Work out the finished part from the listing and answer in its coordinate system (mm). A direction names the side the tool comes from. Round coordinates to 2 decimals unless told otherwise and drop trailing zeros. Order: outer loops, then holes, each group sorted by start corner. A loop starts at its lowest first (then second) coordinate and runs counter-clockwise, first axis right, second up. Notation, with made-up numbers: M 2,-2 L 47,-2 A16 ccw 47,19 Z; hole C -1.5,-35.5 d1. An arc over 180 degrees is marked long. Return JSON: item names as keys, results as strings.
from build123d import *

# Parameters (mm, degrees)
SKETCH1_W                             = 160.4
SKETCH1_H                             = 40
SKETCH1_R                             = 9.5
BOSS_EXTRUDE1_DEPTH                   = 5
TAP_DRILL_FOR_M5_HELICOIL1_AT_2_COUNT = 2
TAP_DRILL_FOR_M5_HELICOIL1_AT_2_PITCH = 20
FILLET1_R                             = 3
M5_CLEARANCE_HOLE1_D                  = 5.5


with BuildPart() as part:
    # Sketch1 → Boss-Extrude1 (new body, symmetric)
    with BuildSketch(Plane(origin=(0, 0, 0), x_dir=(1, 0, 0), z_dir=(0, 1, 0))):
        Rectangle(SKETCH1_W, SKETCH1_H)
        Circle(SKETCH1_R, mode=Mode.SUBTRACT)
    extrude(amount=BOSS_EXTRUDE1_DEPTH, both=True)

    # Sketch4 → Tap Drill for M5 Helicoil1 (revolve, cut)
    with BuildSketch(Plane(origin=(-80.2, 0, -10), x_dir=(0, 0, 1), z_dir=(0, 1, 0))):
        Polygon((0, 0), (0, 31.562237609), (2.6, 30), (2.6, 0), align=None)
    tap_drill_for_m5_helicoil1 = revolve(axis=Axis((-86.55, 0, -10), (1, 0, 0)), mode=Mode.SUBTRACT)

    # Tap Drill for M5 Helicoil1 at 2: Tap Drill for M5 Helicoil1 ×2
    with Locations(*[(0, 0, i * TAP_DRILL_FOR_M5_HELICOIL1_AT_2_PITCH) for i in range(1, TAP_DRILL_FOR_M5_HELICOIL1_AT_2_COUNT)]):
        add(tap_drill_for_m5_helicoil1, mode=Mode.SUBTRACT)

    # Mirror1: Tap Drill for M5 Helicoil1 across plane
    add(tap_drill_for_m5_helicoil1.mirror(Plane(origin=(0, 0, 0), x_dir=(0, 0, 1), z_dir=(1, 0, 0))), mode=Mode.SUBTRACT)

    # Mirror1 copy 1 sketch → Mirror1 copy 1 (revolve, cut)
    with BuildSketch(Plane(origin=(80.2, 0, 10), x_dir=(0, 0, 1), z_dir=(0, 1, 0))):
        Polygon((0, 0), (0, -31.562237609), (2.6, -30), (2.6, 0), align=None)
    revolve(axis=Axis((86.55, 0, 10), (1, 0, 0)), mode=Mode.SUBTRACT)

    # Fillet1
    fillet1_edges = [part.edges().sort_by_distance(p)[0] for p in [
        (-80.2, 0, -20),
        (80.2, 0, -20),
        (80.2, 0, 20),
        (-80.2, 0, 20),
    ]]
    fillet(fillet1_edges, radius=FILLET1_R)

    # M5 Clearance Hole1 (through all)
    with Locations(Plane(origin=(0, 0, -20), x_dir=(-1, 0, 0), z_dir=(0, 0, -1))):
        with Locations((0, 0)):
            Hole(M5_CLEARANCE_HOLE1_D / 2)


solid = part.part
Item 1: Find section A-A (x = 0). Determine the outline of the cut face in (y, z), plus the area to 3 significant figures.
Output:
{"outline": "M -5,-20 L -2.75,-20 L -2.75,-9.5 L -5,-9.5 Z; M -5,9.5 L -2.75,9.5 L -2.75,20 L -5,20 Z; M 2.75,-20 L 5,-20 L 5,-9.5 L 2.75,-9.5 Z; M 2.75,9.5 L 5,9.5 L 5,20 L 2.75,20 Z", "area": "94.5 mm^2"}
Item 2: Find section B-B (z = 0). Determine the outline of the cut face in (x, y), plus the area to 3 significant figures.
Output:
{"outline": "M -80.2,-5 L -9.5,-5 L -9.5,5 L -80.2,5 Z; M 9.5,-5 L 80.2,-5 L 80.2,5 L 9.5,5 Z", "area": "1,410 mm^2"}
Item 3: Find section C-C (x = 56). Determine the outline of the cut face in (y, z), plus the area to 3 significant figures.
Output:
{"outline": "M -5,-20 L 5,-20 L 5,20 L -5,20 Z; hole C 0,-10 d5.2; hole C 0,10 d5.2", "area": "358 mm^2"}
Item 4: Consider line 1 along Y through (x, z) = (0, 14); line 2 along Y through (x, z) = (71, -10); line 3 along X through (y, z) = (-0.25, 0). Determine where each line is inside the solid, lowest interval first. Write a range as [from, to].
Output:
{"line 1": "y = [-5, -2.75], [2.75, 5]", "line 2": "y = [-5, -2.6], [2.6, 5]", "line 3": "x = [-80.2, -9.5], [9.5, 80.2]"}
Item 5: Which of the six approach directions +Z, -Z, +X, -X, +Y, -Y give full straight-line access (tool end or side, diameter ignored) to faces 4 (the cylindrical face through (65.41, -0.78, -7.52)), 5 (the cylindrical face through (-65.41, -0.78, -7.52)), 6 (the cylindrical face through (-79.34, 0.07, 19.1))?
Output:
{"face 4": "+X", "face 5": "-X", "face 6": "+Z, -X, +Y, -Y"}
Item 6: The mould has two halves that part along X. Classify faces 1 (the cylindrical face through (-0.596, -2.685, 14.623)), 2 (the conical face through (48.91, -0.02, 9.55)), 3 (the flat face through (-1, 3, -20)): pulls with the +X half, pulls with the -X half, needs draft (parallel to the pull), parting line crosses it, or undercut.
Output:
{"face 1": "undercut", "face 2": "pulls with the +X half", "face 3": "needs draft"}
Item 7: Each of these flat-tipped pins is pushed along its axis until it touches: pin 1 (2 mm diameter, centred on y = -0.5, z = 10, fed in from -X); pin 2 (3 mm diameter, centred on x = 0, z = -7, fed in from +Y); pin 3 (4.5 mm diameter, centred on y = 0, z = 10, fed in from -X). Where does it stop, or does it pass through?
Output:
{"pin 1": "stops at x = -49.54", "pin 2": "passes through", "pin 3": "stops at x = -49.99"}
